from build123d import *

# Parameters (mm, degrees)
ESQUISSE1_R                  = 11.5
ESQUISSE1_R_2                = 3.175
BOSS_EXTRU_1_DEPTH           = 27
ESQUISSE2_R                  = 11.5
ESQUISSE2_R_2                = 9.17
ENL_V_MAT_EXTRU_1_DEPTH      = 16
ENL_V_START                  = 16
ENL_V_MAT_EXTRU_2_DEPTH      = 16
R_P_TITION_CIRCULAIRE1_COUNT = 20
ESQUISSE4_R                  = 2
ENL_V_MAT_EXTRU_3_DEPTH      = 16
R_P_TITION_CIRCULAIRE2_COUNT = 2
R_P_TITION_CIRCULAIRE2_ANGLE = 90
ESQUISSE5_R                  = 7.5
ENL_V_MAT_EXTRU_4_DEPTH      = 0.5
CHANFREIN1_SIZE              = 0.25


with BuildPart() as part:
    # Esquisse1 → Boss.-Extru.1 (new body)
    with BuildSketch(Plane.XY):
        Circle(ESQUISSE1_R)
        Circle(ESQUISSE1_R_2, mode=Mode.SUBTRACT)
    extrude(amount=BOSS_EXTRU_1_DEPTH)

    # Esquisse2 → Enlèv. mat.-Extru.1 (cut)
    with BuildSketch(Plane(origin=(0, 0, 1.5), x_dir=(-1, 0, 0), z_dir=(0, 0, -1))):
        Circle(ESQUISSE2_R)
        Circle(ESQUISSE2_R_2, mode=Mode.SUBTRACT)
    extrude(amount=-ENL_V_MAT_EXTRU_1_DEPTH, mode=Mode.SUBTRACT)

    # Esquisse3 → Enlèv. mat.-Extru.2 (cut)
    with BuildSketch(Plane(origin=(0, 0, 17.5), x_dir=(-1, 0, 0), z_dir=(0, 0, -1)).offset(ENL_V_START)):
        with BuildLine():
            ThreePointArc((-1.5, 9.046485505), (-0.88232463, 8.905445978), (-0.541125011, 8.371594096))
            ThreePointArc((-0.541125011, 8.371594096), (0, 7.92), (0.541125011, 8.371594096))
            ThreePointArc((0.541125011, 8.371594096), (0.88232463, 8.905445978), (1.5, 9.046485505))
            ThreePointArc((1.5, 9.046485505), (0, 9.17), (-1.5, 9.046485505))
        make_face()
    enl_v_mat_extru_2 = extrude(amount=-ENL_V_MAT_EXTRU_2_DEPTH, mode=Mode.SUBTRACT)

    # Répétition circulaire1: Enlèv. mat.-Extru.2 ×20 about axis
    r_p_tition_circulaire1_axis = Axis((0, 0, 0), (0, 0, 1))
    for i in range(1, R_P_TITION_CIRCULAIRE1_COUNT):
        add(enl_v_mat_extru_2.rotate(r_p_tition_circulaire1_axis, i * 360 / R_P_TITION_CIRCULAIRE1_COUNT), mode=Mode.SUBTRACT)

    # Esquisse4 → Enlèv. mat.-Extru.3 (cut)
    with BuildSketch(Plane(origin=(0, 0, 0), x_dir=(1, 0, 0), z_dir=(0, 1, 0))):
        with Locations(Location((0, -22.25, 0), (0, 0, 270))):
            Circle(ESQUISSE4_R)
    enl_v_mat_extru_3 = extrude(amount=-ENL_V_MAT_EXTRU_3_DEPTH, mode=Mode.SUBTRACT)

    # Répétition circulaire2: Enlèv. mat.-Extru.3 ×2 about axis
    r_p_tition_circulaire2_axis = Axis((0, 0, 27), (0, 0, 1))
    for i in range(1, R_P_TITION_CIRCULAIRE2_COUNT):
        add(enl_v_mat_extru_3.rotate(r_p_tition_circulaire2_axis, i * R_P_TITION_CIRCULAIRE2_ANGLE / (R_P_TITION_CIRCULAIRE2_COUNT - 1)), mode=Mode.SUBTRACT)

    # Esquisse5 → Enlèv. mat.-Extru.4 (cut)
    with BuildSketch(Plane(origin=(0, 0, 0), x_dir=(-1, 0, 0), z_dir=(0, 0, -1))):
        Circle(ESQUISSE5_R)
    enl_v_mat_extru_4 = extrude(amount=-ENL_V_MAT_EXTRU_4_DEPTH, mode=Mode.SUBTRACT)

    # Symétrie1: Enlèv. mat.-Extru.4 across plane
    add(enl_v_mat_extru_4.mirror(Plane(origin=(0, 0, 13.5), x_dir=(1, 0, 0), z_dir=(0, 0, -1))), mode=Mode.SUBTRACT)

    # Chanfrein1
    chanfrein1_edges = [part.edges().sort_by_distance(p)[0] for p in [
        (-11.5, 0, 17.5),
        (-11.5, 0, 1.5),
        (-3.175, 0, 0.5),
        (7.5, 0, 0),
        (-11.5, 0, 0),
        (7.5, 0, 27),
        (-3.175, 0, 26.5),
        (-11.5, 0, 27),
    ]]
    chamfer(chanfrein1_edges, length=CHANFREIN1_SIZE)


solid = part.part
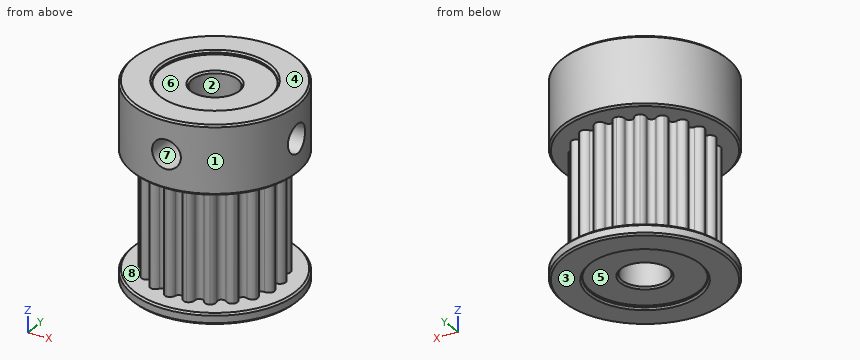
Work out the finished part from the listing and answer in its coordinate system (mm). Face numbers are marked on the shaded views. A direction names the side the tool comes from. Give positions to 0.01 mm unless a question says otherwise; leave off trailing zeros. Return JSON: item names as keys, results as strings.
Q1. Find section B-B, the plane y = -9.75. State how many separate pieces and enclosed holes the cut face has, and give its area (3 significant figures).
Answer below:
{"separate pieces": "2", "enclosed holes": "1", "area": "121 mm^2"}
Q2. The mould has two halves that part along Y. Classify the marked faces 1, 2 and 3: pulls with the +Y half, pulls with the -Y half, needs draft (parallel to the pull), parting line crosses it, or undercut.
Answer below:
{"face 1": "parting line crosses it", "face 2": "undercut", "face 3": "needs draft"}
Q3. Which of the six approach directions +Z, -Z, +X, -X, +Y, -Y give full straight-line access (tool end or side, diameter ignored) to the marked faces 4, 5, 6, 7 and 8?
Answer below:
{"face 4": "+Z, +X, -X, +Y, -Y", "face 5": "-Z", "face 6": "+Z", "face 7": "-Y", "face 8": "none"}
Q4. Find the intervals of material crossed by line 1 along Z through (x, y) = (0, -8); line 2 along Z through (x, y) = (9, 5.75); line 3 along Y through (x, z) = (0, 20) (3 decimals), in increasing order. Write a range as [from, to].
Answer below:
{"line 1": "z = [0, 1.5], [17.5, 20.25], [24.25, 27]", "line 2": "z = [0, 1.5], [17.5, 27]", "line 3": "y = [-11.5, -3.175], [3.175, 11.5]"}
Q5. Each of these flat-tipped pins is pushed along its axis until it touches: pin 1 (5 mm diameter, centred on y = -4.5, z = 23, fed in from +X); pin 2 (10 mm diameter, centred on y = -9, z = 10.5, fed in from -X); pin 3 (7.5 mm diameter, centred on x = -3, y = 0, fed in from -Z). Where does it stop, or does it pass through?
Answer below:
{"pin 1": "stops at x = 11.32", "pin 2": "stops at x = -8.22", "pin 3": "stops at z = 0.5"}
